Design review of the part built by this model. Coordinates are the model's own, in mm. Give positions to 0.01 mm unless a question says otherwise; leave off trailing zeros. Order: outer loops, then holes, each group sorted by start corner. A loop starts at its lowest first (then second) coordinate and runs counter-clockwise, first axis right, second up. Notation, with made-up numbers: (-26, 63) -> (14, 63) arc R25 cw to (14, 92) -> close; hole circle Ø11 at (57, -9). An arc over 180 degrees is marked (long way). One line per item, written item: value. Start each with the question number.
1) For pin 1 (10 mm diameter, centred on x = 463.5, y = 26.5, fed in from +Z); pin 2 (6.5 mm diameter, centred on x = 88.9, y = 12.7, fed in from -Z); pin 3 (3 mm diameter, centred on x = 479.5, z = -2.5, fed in from -Y); pin 4 (2 mm diameter, centred on x = 349.5, z = -1, fed in from +Y), all flat-tipped, find the tip position at first contact; note any pin that passes through.
2) Wall thickness on line 1 along Y through (x, z) = (317.5, -3); line 2 along Y through (x, z) = (12.7, -1.5); line 3 along Y through (x, z) = (295, -1): over which ranges is each line inside the solid? List them lowest first. Write a range as from..to.
3) Consider section A-A (z = -2). State how many separate pieces and enclosed holes the cut face has, plus the area to 3 significant figures.
4) Consider section B-B (x = 57). State the section outline as (y, z) points.
from build123d import *

# Parameters (mm, degrees)
SKETCH1_R                                          = 2.4892
BOSS_EXTRUDE1_DEPTH                                = 6.477
FILLET2_R                                          = 6.35
CSK_FOR_10_FLAT_HEAD_MACHINE_SCREW_100_D           = 5.1054
CSK_FOR_10_FLAT_HEAD_MACHINE_SCREW_100_CSINK_D     = 9.779
CSK_FOR_10_FLAT_HEAD_MACHINE_SCREW_100_CSINK_ANGLE = 100
LPATTERN1_COUNT                                    = 8
LPATTERN1_PITCH                                    = 76.2
FILLET3_R                                          = 3.175


with BuildPart() as part:
    # Sketch1 → Boss-Extrude1 (new body)
    with BuildSketch(Plane.XY):
        Polygon((0, 0), (40.53078, 0), (417.140898, 0), (417.140898, -9.525), (442.540898, -9.525), (442.540898, 0), (584.2, 0), (584.2, 25.4), (40.53078, 25.4), (40.53078, 34.925), (15.13078, 34.925), (15.13078, 25.4), (0, 25.4), align=None)
        with Locations((577.85, 6.35)):
            Circle(SKETCH1_R, mode=Mode.SUBTRACT)
    extrude(amount=BOSS_EXTRUDE1_DEPTH)

    # Fillet2
    fillet2_edges = [part.edges().sort_by_distance(p)[0] for p in [
        (0, 0, 3.2385),
        (0, 25.4, 3.2385),
        (584.2, 25.4, 3.2385),
        (584.2, 0, 3.2385),
    ]]
    fillet(fillet2_edges, radius=FILLET2_R)

    # CSK for #10 Flat Head Machine Screw (100)1 (through all)
    with Locations(Plane.XY.offset(6.477)):
        with Locations((546.1, 12.7)):
            csk_for_10_flat_head_machine_screw_100 = CounterSinkHole(CSK_FOR_10_FLAT_HEAD_MACHINE_SCREW_100_D / 2, CSK_FOR_10_FLAT_HEAD_MACHINE_SCREW_100_CSINK_D / 2, counter_sink_angle=CSK_FOR_10_FLAT_HEAD_MACHINE_SCREW_100_CSINK_ANGLE)

    # LPattern1: CSK for #10 Flat Head Machine Screw (100)1 ×8
    with Locations(*[(-i * LPATTERN1_PITCH, 0, 0) for i in range(1, LPATTERN1_COUNT)]):
        add(csk_for_10_flat_head_machine_screw_100, mode=Mode.SUBTRACT)


with BuildPart() as body_2:
    # Mirror2: mirrored copy
    add(part.part.mirror(Plane.XY))

    # Fillet3
    fillet3_edges = [body_2.edges().sort_by_distance(p)[0] for p in [
        (442.540898, -9.525, -3.2385),
        (417.140898, -9.525, -3.2385),
        (417.140898, 0, -3.2385),
        (15.13078, 25.4, -3.2385),
        (15.13078, 34.925, -3.2385),
        (40.53078, 34.925, -3.2385),
        (40.53078, 25.4, -3.2385),
        (442.540898, 0, -3.2385),
    ]]
    fillet(fillet3_edges, radius=FILLET3_R)


solid = body_2.part
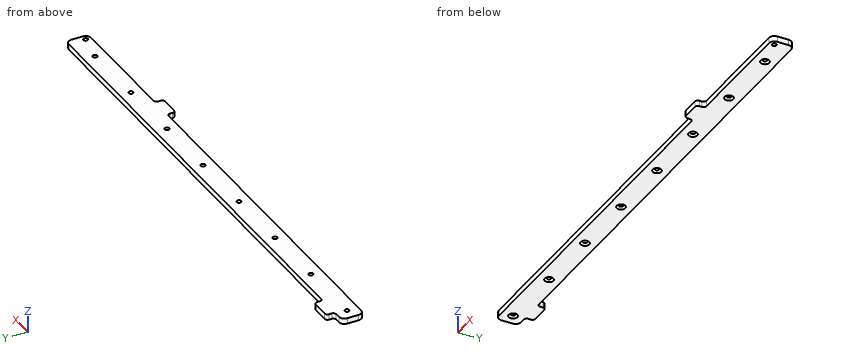
Checked values:
1. pin 1: stops at z = 0
1. pin 2: stops at z = -5.1
1. pin 3: stops at y = 0
1. pin 4: stops at y = 25.4
2. line 1: y = 0..10.15, 15.25..25.4
2. line 2: y = 0..10.15, 15.25..25.49
2. line 3: y = 0..25.4
3. separate pieces: 1
3. enclosed holes: 9
3. area: 15,100 mm^2
4. outline: (0, -6.48) -> (25.4, -6.48) -> (25.4, 0) -> (0, 0) -> close
